Input: part model. Units: mm. Frame: model coordinates. Round coordinates to 2 decimals unless told otherwise and drop trailing zeros. Loops run counter-clockwise (first coordinate to the right, second up) from the corner with the lowest first, then second, coordinate; pieces in that order, holes last.
(1) Cut plane C-C, the plane z = -14.5. Output: boundary loops of the cut face in (x, y).
(2) Cut plane A-A, the plane y = 277. Output: boundary loops of the cut face in (x, z).
(3) Cut plane D-D, the plane y = 369.5. Output: boundary loops of the cut face in (x, z).
(4) First-contact query: pin 1 Ø5 at (x, z) = (225, -14) entering from +Y; pin 2 Ø1.5 at (x, z) = (353.5, -11.5) entering from -Y; pin 3 Ø10 at (x, z) = (211.5, -2.5) entering from -Y; pin 4 Ø3 at (y, z) = (175, -17) entering from +X. Flat tips, straight axial feed; report the tip coordinate or a pass-through.
(5) Line query: line 1 (Z direction, x = 38, y = 160.5); line 2 (Y direction, x = 324.5, z = -12). Output: solid intervals per line, ascending.
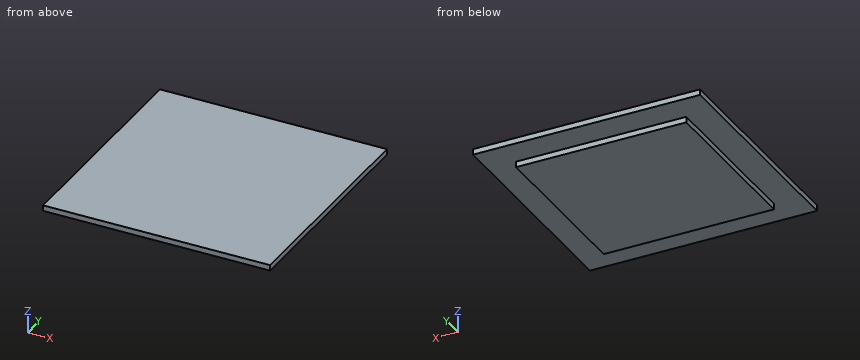
from build123d import *

# Parameters (mm, degrees)
BOX004_W     = 300
BOX004_H     = 300
BOX004_DEPTH = 10
BOX003_W     = 400
BOX003_H     = 400
BOX003_DEPTH = 10


with BuildPart() as cube003:
    # Box004 → Box004 (new body)
    with BuildSketch(Plane(origin=(50, 50, -20), x_dir=(1, 0, 0), z_dir=(0, 0, 1))):
        with Locations((150, 150)):
            Rectangle(BOX004_W, BOX004_H)
    extrude(amount=BOX004_DEPTH)


with BuildPart() as w_plate:
    # Box003 → Box003 (new body)
    with BuildSketch(Plane.XY.offset(-10)):
        with Locations((200, 200)):
            Rectangle(BOX003_W, BOX003_H)
    extrude(amount=BOX003_DEPTH)

    # Fusion: union Cube003
    add(cube003.part)


solid = w_plate.part
Reported:
1. outline: (50, 50) - (350, 50) - (350, 350) - (50, 350) - close
2. outline: (0, -10) - (50, -10) - (50, -20) - (350, -20) - (350, -10) - (400, -10) - (400, 0) - (0, 0) - close
3. outline: (0, -10) - (400, -10) - (400, 0) - (0, 0) - close
4. pin 1: stops at y = 350
4. pin 2: passes through
4. pin 3: stops at y = 0
4. pin 4: stops at x = 350
5. line 1: z = -10 to 0
5. line 2: y = 50 to 350
